from build123d import *

# Parameters (mm, degrees)
SKETCH1_R           = 9.525
SKETCH1_R_2         = 2.54
SKETCH1_R_3         = 14.2875
BOSS_EXTRUDE1_DEPTH = 6.35
FILLET2_R           = 6.35


with BuildPart() as part:
    # Sketch1 → Boss-Extrude1 (new body)
    with BuildSketch(Plane.XY):
        with BuildLine():
            Line((0, 0), (0, 39.37))
            Line((0, 39.37), (40.53078, 39.37))
            Line((40.53078, 39.37), (548.64, 39.37))
            Line((548.64, 39.37), (548.64, 77.47))
            ThreePointArc((548.64, 77.47), (579.12, 107.95), (609.6, 77.47))
            Line((609.6, 77.47), (609.6, 0))
            Line((609.6, 0), (0, 0))
        make_face()
        with Locations((579.12, 77.47)):
            Circle(SKETCH1_R, mode=Mode.SUBTRACT)
        with Locations((579.12, 102.87)):
            Circle(SKETCH1_R_2, mode=Mode.SUBTRACT)
        with Locations((591.82, 99.467045256)):
            Circle(SKETCH1_R_2, mode=Mode.SUBTRACT)
        with Locations((601.117045256, 90.17)):
            Circle(SKETCH1_R_2, mode=Mode.SUBTRACT)
        with Locations((604.52, 77.47)):
            Circle(SKETCH1_R_2, mode=Mode.SUBTRACT)
        with Locations((601.117045256, 64.77)):
            Circle(SKETCH1_R_2, mode=Mode.SUBTRACT)
        with Locations((591.82, 55.472954744)):
            Circle(SKETCH1_R_2, mode=Mode.SUBTRACT)
        with Locations((579.12, 52.07)):
            Circle(SKETCH1_R_2, mode=Mode.SUBTRACT)
        with Locations((566.42, 55.472954744)):
            Circle(SKETCH1_R_2, mode=Mode.SUBTRACT)
        with Locations((557.122954744, 64.77)):
            Circle(SKETCH1_R_2, mode=Mode.SUBTRACT)
        with Locations((553.72, 77.47)):
            Circle(SKETCH1_R_2, mode=Mode.SUBTRACT)
        with Locations((557.122954744, 90.17)):
            Circle(SKETCH1_R_2, mode=Mode.SUBTRACT)
        with Locations((566.42, 99.467045256)):
            Circle(SKETCH1_R_2, mode=Mode.SUBTRACT)
        with Locations((579.12, 23.378627903)):
            Circle(SKETCH1_R_3, mode=Mode.SUBTRACT)
    extrude(amount=BOSS_EXTRUDE1_DEPTH)

    # Fillet2
    fillet2_edges = [part.edges().sort_by_distance(p)[0] for p in [
        (609.6, 0, 3.175),
        (0, 0, 3.175),
        (0, 39.37, 3.175),
        (548.64, 39.37, 3.175),
    ]]
    fillet(fillet2_edges, radius=FILLET2_R)


solid = part.part
Input: part model. Units: mm. Frame: model coordinates. Coordinates: 2 decimals unless noted, no trailing zeros. Loops run counter-clockwise (first coordinate to the right, second up) from the corner with the lowest first, then second, coordinate; pieces in that order, holes last.
(1) Pull-direction query (Y, two-part tool) for faces 1 (the face through (567.782, 14.685, 3.131)), 2 (the face through (588.205, 80.331, 3.131)), 3 (the face through (329, 30, 6.35)), 4 (the face through (578.45, 107.943, 3.131)); classes: released by +Y, released by -Y, zero draft, split by the parting line, or undercut.
(2) Section A-A on z = 2.5. Count the separate pieces of the cut face and the enclosed holes in it, then the cut area to 3 significant figures.
(3) Section B-B on x = 275. Return the cut outline in (y, z), then the cut area to 3 significant figures.
(4) Material intervals for probe 1 along Y at (x, z) = (579.12, 2) (3 decimals); probe 2 along Y at (x, z) = (591.82, 1.75); probe 3 along X at (y, z) = (52, 5), sorted ascending.
(5) First-contact query: pin 1 Ø3 at (y, z) = (86, 3) entering from -X. Flat tip, straight axial feed; report the tip coordinate or a pass-through.
Data:
1. face 1: undercut
1. face 2: undercut
1. face 3: zero draft
1. face 4: released by +Y
2. separate pieces: 1
2. enclosed holes: 14
2. area: 26,600 mm2
3. outline: (0, 0) - (39.37, 0) - (39.37, 6.35) - (0, 6.35) - close
3. area: 250 mm2
4. probe 1: y = 0 to 9.091, 37.666 to 49.53, 54.61 to 67.945, 86.995 to 100.33, 105.41 to 107.95
4. probe 2: y = 0 to 16.83, 29.92 to 52.93, 58.01 to 96.93, 102.01 to 105.18
4. probe 3: x = 548.64 to 576.58, 581.66 to 609.6
5. pin 1: stops at x = 549.46
